Read the model definition and answer for the solid it produces. Units are mm, in the model's axes. A direction names the side the tool comes from. Coordinates: 2 decimals unless noted, no trailing zeros. Order: outer loops, then holes, each group sorted by start corner. A loop starts at its lowest first (then second) coordinate and runs counter-clockwise, first axis right, second up.
Autodesk Inventor part; units mm, degrees
ref_plane "YZ Plane" through (0, 0, 0) normal (1, 0, 0) x (0, 1, 0)
ref_plane "XZ Plane" through (0, 0, 0) normal (0, 1, 0) x (-1, 0, 0)
ref_plane "XY Plane" through (0, 0, 0) normal (0, 0, 1) x (1, 0, 0)
sketch "Эскиз1" plane through (0, 0, 0) normal (0, 0, 1) x (1, 0, 0)
  line L0 (0, 31) -> (0, 45)
  line L1 (0, 45) -> (6, 45)
  line L2 (6, 45) -> (6.5, 44.5)
  line L3 (6.5, 44.5) -> (11.5, 44.5)
  line L4 (11.5, 44.5) -> (11.5, 48)
  line L5 (11.5, 48) -> (17.5, 48)
  line L6 (17.5, 48) -> (17.5, 45)
  line L7 (17.5, 39) -> (10, 39)
  line L8 (10, 39) -> (10, 36)
  line L9 (10, 36) -> (2, 36)
  line L10 (2, 36) -> (2, 31)
  line L11 (2, 31) -> (0, 31)
  line L12 (0, 0) -> (122.1011, 0) construction
  line L13 (17.5, 45) -> (20.55, 45)
  line L14 (20.55, 45) -> (20.55, 39)
  line L15 (20.55, 39) -> (17.5, 39)
  dimension "d0" = 90
  dimension "d1" = 72
  dimension "d2" = 5
  dimension "d4" = 5
  dimension "d5" = 6
  dimension "d7" = 45
  dimension "d8" = 0.5
  dimension "d9" = 9
  dimension "d10" = 6
  dimension "d12" = 2
  dimension "d19" = 96
  dimension "d20" = 10
  dimension "d24" = 3.05
revolve "Вращение1" add sketch "Эскиз1" angle 360 about axis through (0, 0, 0) along (1, 0, 0)
fillet "Сопряжение1" radius 1.6 2 edges at (6.5, -44.5, 0) (11.5, -44.5, 0)
chamfer "Фаска1" distance 1 angle 45 2 edges at (0, -45, 0) (17.5, -39, 0)
properties part number "Крышка тих_выход"
Q1. The part is cut by section B-B, the plane x = 15.75. Determine the outline of the cut face in (y, z).
Q2. Determine the mould class of faces 1 (the flat face through (17.5, 14, 43)), 2 (the cylindrical face through (0.986, -4.036, -30.736)), 3 (the flat face through (2, 16, 27)), 4 (the cylindrical face through (3.535, 20.765, -39.923)) for opening direction Z: +Z half, -Z half, draft (parallel to the pull), parting line (faces both ways), or undercut.
Q3. Straight lines are drawn through the part: L1, parallel to Z at x = 15.5, y = 0; L2, parallel to Z at x = 1.25, y = 0; L3, parallel to Y at x = 16.25, z = 8.5. For each, find the intervals that lie inside material, in ascending order.
Q4. Each of these flat-tipped pins is pushed along its axis until it touches: P1, Ø4, axis at y = 1, z = 31, coming from the +X side; P2, Ø1, axis at x = 16.5, z = -9, coming from the -Y side; P3, Ø3, axis at x = 13.5, z = -38, coming from the -Y side. Where does it stop, or does it pass through?
Q5. Which of the six approach directions +Z, -Z, +X, -X, +Y, -Y give full straight-line access (tool end or side, diameter ignored) to faces 5 (the cylindrical face through (14.542, -47.954, 2.11)), 6 (the flat face through (11.5, -43, 18)), 7 (the cylindrical face through (19.046, 20.765, -39.923)), 8 (the flat face through (20.55, -14, 37)), 9 (the cylindrical face through (8.55, -35.31, -27.08))?
Q6. The part is cut by section A-A, the plane x = 3.25. Determine the outline of the cut face in (y, z), then the cut area to 3 significant figures.
Computed values:
1. outline: circle Ø96 at (0, 0); hole circle Ø78 at (0, 0)
2. face 1: draft
2. face 2: undercut
2. face 3: undercut
2. face 4: parting line
3. L1: z = -48 to -39, 39 to 48
3. L2: z = -45 to -31, 31 to 45
3. L3: y = -47.24 to -38.06, 38.06 to 47.24
4. P1: stops at x = 2
4. P2: stops at y = -47.24
4. P3: stops at y = -31.17
5. face 5: +X, -X
5. face 6: -X
5. face 7: +X
5. face 8: +Z, -Z, +X, +Y, -Y
5. face 9: none
6. outline: circle Ø90 at (0, 0); hole circle Ø72 at (0, 0)
6. area: 2,290 mm2
